The figure shows three views and two pictorial views of one solid part (mm, origin at its lowest corner). Answer the questions. Round coordinates to 2 decimals unless told otherwise and drop trailing zeros. Write each loop counter-clockwise with the first axis right and the second up, starting at its lowest first coordinate (ties: lowest second). Pieces come first, ordered by that corner, then holes. Notation, with made-up numbers: M 31.5,-30.75 L 71.5,-30.75 A21 ccw 71.5,-21.75 Z; hole C -36.75,-9.75 d10. An arc over 180 degrees is marked long. Use one line per item in the form item = value. Start each with the question number.
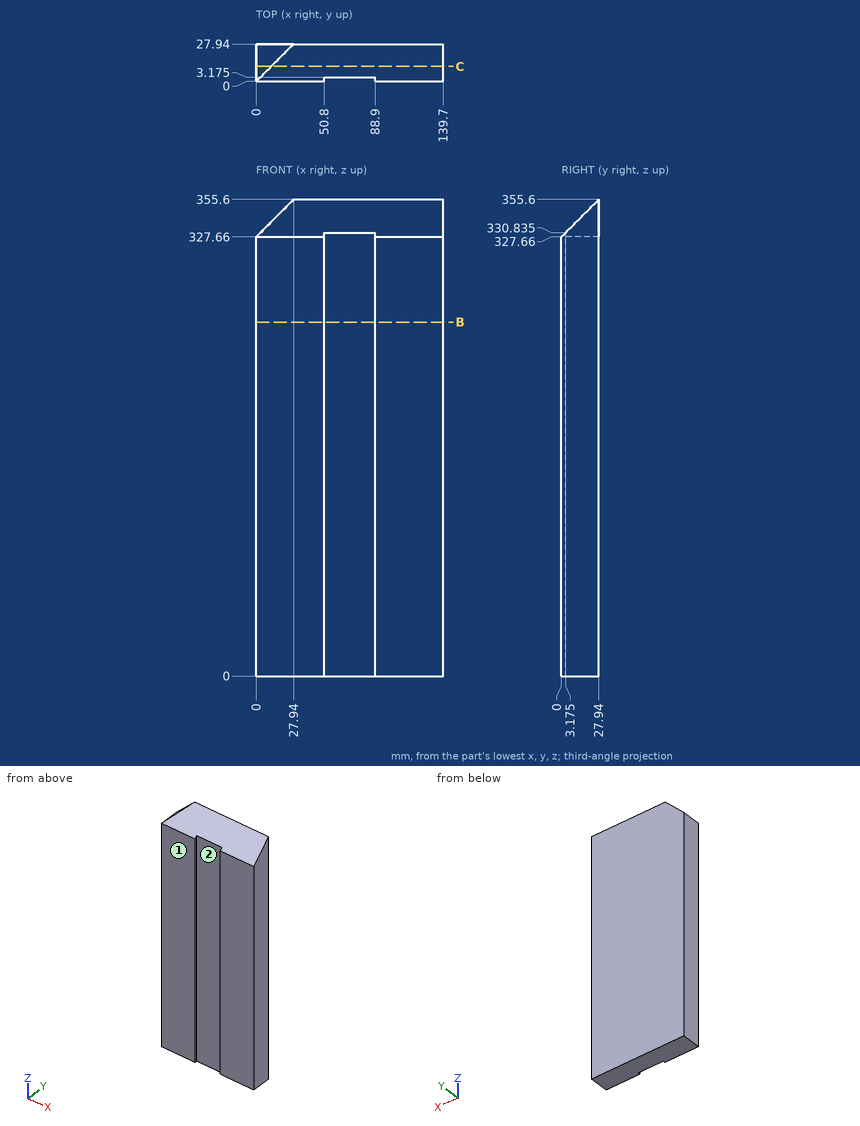
Q1. Straight lines are drawn through the part: line 1 (Z direction, x = 28, y = 3.25); line 2 (Y direction, x = 70.5, z = 74.5) (3 decimals); line 3 (Z direction, x = 121, y = 13). For each, find the intervals that lie inside material, in ascending order. Write a range as [from, to].
Q2. Each of these flat-tipped pins is pushed along its axis until it touches: pin 1 Ø6 at (x, y) = (23, 17) entering from +Z; pin 2 Ø11.5 at (x, z) = (70, 94) entering from -Y (3 decimals); pin 3 Ø1 at (x, y) = (69.5, 3.5) entering from +Z. Where does it stop, or does it pass through?
Q3. Find section B-B on z = 264. Write down the section's boundary in (x, y) (3 decimals).
Q4. For a pull along X with two mould halves and no side action, classify the marked faces 1 and 2 as +X half, -X half, draft (parallel to the pull), parting line (faces both ways), or undercut.
Q5. Find section C-C on y = 11.25. Write down the section's boundary in (x, z), and give its area (3 significant figures).
Response:
q1.line_1 = [0, 330.91]
q1.line_2 = [3.175, 27.94]
q1.line_3 = [0, 340.66]
q2.pin_1 = 347.66
q2.pin_2 = 3.175
q2.pin_3 = 331.66
q3.outline = M 0,0 L 50.8,0 L 50.8,3.175 L 88.9,3.175 L 88.9,0 L 139.7,0 L 139.7,27.94 L 0,27.94 Z
q4.face_1 = draft
q4.face_2 = undercut
q5.outline = M 0,0 L 139.7,0 L 139.7,338.91 L 11.25,338.91 L 0,327.66 Z
q5.area = 47,300 mm²
